The model under review builds one solid part; all positions refer to its coordinate system, in mm. Coordinates: 2 decimals unless noted, no trailing zeros. Order: outer loops, then holes, each group sorted by start corner. A loop starts at its lowest first (then second) coordinate and runs counter-clockwise, first axis right, second up.
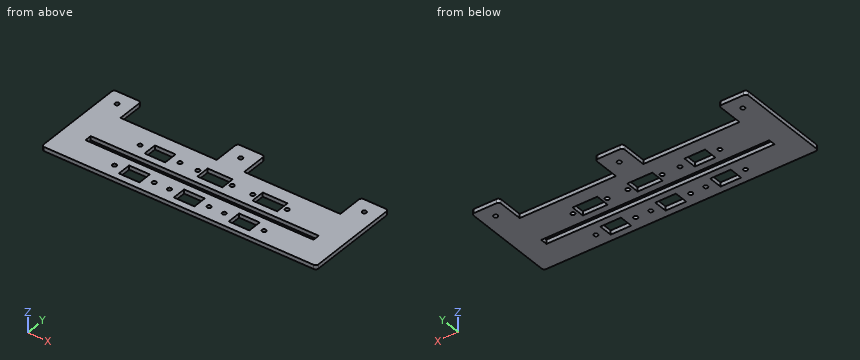
```python
from build123d import *

# Parameters (mm, degrees)
SKETCH_1_W           = 200
SKETCH_1_H           = 70
EXTRUDE_1_DEPTH      = 3
SKETCH_2_W           = 70
SKETCH_2_H           = 20
CUT_EXTRUDE_1_DEPTH  = 3
SKETCH_4_W           = 70
SKETCH_4_H           = 20
CUT_EXTRUDE_2_DEPTH  = 3
SKETCH_5_W           = 166
SKETCH_5_H           = 5
CUT_EXTRUDE_3_DEPTH  = 3
CUT_EXTRUDE_8_DEPTH  = 3
SKETCH_7_R           = 1.5
CUT_EXTRUDE_9_DEPTH  = 3
SKETCH_8_W           = 15
SKETCH_8_H           = 10
CUT_EXTRUDE_10_DEPTH = 3
SKETCH_9_W           = 15
SKETCH_9_H           = 10
SKETCH_9_W_2         = 18
SKETCH_9_W_3         = 18.2
CUT_EXTRUDE_11_DEPTH = 3
SKETCH_10_R          = 1.5
CUT_EXTRUDE_12_DEPTH = 3


with BuildPart() as part:
    # ｽｹｯﾁ1 → ﾎﾞｽ - 押し出し1 (new body)
    with BuildSketch(Plane.XY):
        Rectangle(SKETCH_1_W, SKETCH_1_H)
    extrude(amount=EXTRUDE_1_DEPTH)

    # ｽｹｯﾁ2 → ｶｯﾄ - 押し出し1 (cut)
    with BuildSketch(Plane.XY.offset(3)):
        with Locations((-45, 25)):
            Rectangle(SKETCH_2_W, SKETCH_2_H)
    extrude(amount=-CUT_EXTRUDE_1_DEPTH, mode=Mode.SUBTRACT)

    # ｽｹｯﾁ4 → ｶｯﾄ - 押し出し2 (cut)
    with BuildSketch(Plane.XY.offset(3)):
        with Locations((45, 25)):
            Rectangle(SKETCH_4_W, SKETCH_4_H)
    extrude(amount=-CUT_EXTRUDE_2_DEPTH, mode=Mode.SUBTRACT)

    # ｽｹｯﾁ5 → ｶｯﾄ - 押し出し3 (cut)
    with BuildSketch(Plane.XY.offset(3)):
        with Locations((0, -12.5)):
            Rectangle(SKETCH_5_W, SKETCH_5_H)
    extrude(amount=-CUT_EXTRUDE_3_DEPTH, mode=Mode.SUBTRACT)

    # ｽｹｯﾁ6 → ｶｯﾄ - 押し出し8 (cut)
    with BuildSketch(Plane.XY.offset(3)):
        with BuildLine():
            ThreePointArc((-98, -35), (-99.414213562, -34.414213562), (-100, -33))
            Line((-100, -33), (-100, -35))
            Line((-100, -35), (-98, -35))
        make_face()
        with BuildLine():
            Line((-100, 35), (-100, 33))
            ThreePointArc((-100, 33), (-99.414213562, 34.414213562), (-98, 35))
            Line((-98, 35), (-100, 35))
        make_face()
        with BuildLine():
            ThreePointArc((100, -33), (99.414213562, -34.414213562), (98, -35))
            Line((98, -35), (100, -35))
            Line((100, -35), (100, -33))
        make_face()
        with BuildLine():
            Line((-80, 35), (-82, 35))
            ThreePointArc((-82, 35), (-80.585786438, 34.414213562), (-80, 33))
            Line((-80, 33), (-80, 35))
        make_face()
        with BuildLine():
            ThreePointArc((98, 35), (99.414213562, 34.414213562), (100, 33))
            Line((100, 33), (100, 35))
            Line((100, 35), (98, 35))
        make_face()
        with BuildLine():
            ThreePointArc((80, 33), (80.585786438, 34.414213562), (82, 35))
            Line((82, 35), (80, 35))
            Line((80, 35), (80, 33))
        make_face()
        with BuildLine():
            Line((-10, 35), (-10, 33))
            ThreePointArc((-10, 33), (-9.414213562, 34.414213562), (-8, 35))
            Line((-8, 35), (-10, 35))
        make_face()
        with BuildLine():
            Line((10, 35), (8, 35))
            ThreePointArc((8, 35), (9.414213562, 34.414213562), (10, 33))
            Line((10, 33), (10, 35))
        make_face()
    extrude(amount=-CUT_EXTRUDE_8_DEPTH, mode=Mode.SUBTRACT)

    # ｽｹｯﾁ7 → ｶｯﾄ - 押し出し9 (cut)
    with BuildSketch(Plane.XY.offset(3)):
        with Locations((-90, 25)):
            Circle(SKETCH_7_R)
        with Locations((0, 25)):
            Circle(SKETCH_7_R)
        with Locations((90, 25)):
            Circle(SKETCH_7_R)
    extrude(amount=-CUT_EXTRUDE_9_DEPTH, mode=Mode.SUBTRACT)

    # ｽｹｯﾁ8 → ｶｯﾄ - 押し出し10 (cut)
    with BuildSketch(Plane.XY.offset(3)):
        with Locations((40, -25)):
            Rectangle(SKETCH_8_W, SKETCH_8_H)
        with Locations((0, -25)):
            Rectangle(SKETCH_8_W, SKETCH_8_H)
        with Locations((-40, -25)):
            Rectangle(SKETCH_8_W, SKETCH_8_H)
    extrude(amount=-CUT_EXTRUDE_10_DEPTH, mode=Mode.SUBTRACT)

    # ｽｹｯﾁ9 → ｶｯﾄ - 押し出し11 (cut)
    with BuildSketch(Plane.XY.offset(3)):
        with Locations((-40, 0)):
            Rectangle(SKETCH_9_W, SKETCH_9_H)
        with Locations((40, 0)):
            Rectangle(SKETCH_9_W_2, SKETCH_9_H)
        Rectangle(SKETCH_9_W_3, SKETCH_9_H)
    extrude(amount=-CUT_EXTRUDE_11_DEPTH, mode=Mode.SUBTRACT)

    # ｽｹｯﾁ10 → ｶｯﾄ - 押し出し12 (cut)
    with BuildSketch(Plane.XY.offset(3)):
        with Locations((-54.5, 0)):
            Circle(SKETCH_10_R)
        with Locations((-25.5, 0)):
            Circle(SKETCH_10_R)
        with Locations((-12.5, 0)):
            Circle(SKETCH_10_R)
        with Locations((12.5, 0)):
            Circle(SKETCH_10_R)
        with Locations((27.5, 0)):
            Circle(SKETCH_10_R)
        with Locations((52.5, 0)):
            Circle(SKETCH_10_R)
        with Locations((54.5, -25)):
            Circle(SKETCH_10_R)
        with Locations((25.5, -25)):
            Circle(SKETCH_10_R)
        with Locations((14.5, -25)):
            Circle(SKETCH_10_R)
        with Locations((-14.5, -25)):
            Circle(SKETCH_10_R)
        with Locations((-25.5, -25)):
            Circle(SKETCH_10_R)
        with Locations((-54.5, -25)):
            Circle(SKETCH_10_R)
    extrude(amount=-CUT_EXTRUDE_12_DEPTH, mode=Mode.SUBTRACT)


solid = part.part
```
(1) We need section C-C, the plane z = 0.7. Count the separate pieces of the cut face and the enclosed holes in it, and give its area (3 significant figures).
A:
separate pieces: 1
enclosed holes: 22
area: 9,300 mm2
(2) For pin 1 Ø1.8 at (x, y) = (-25.5, -25) entering from -Z, flat-tipped, find the tip position at first contact; note if it passes through.
A:
pin 1: passes through
(3) We need section B-B, the plane x = -20.5. Write out the cut boundary in (y, z), and give its area (3 significant figures).
A:
outline: (-35, 0) - (-15, 0) - (-15, 3) - (-35, 3) - close; (-10, 0) - (15, 0) - (15, 3) - (-10, 3) - close
area: 135 mm2
(4) We need section A-A, the plane y = 21.5. Write out the cut boundary in (x, z), and give its area (3 significant figures).
A:
outline: (-100, 0) - (-80, 0) - (-80, 3) - (-100, 3) - close; (-10, 0) - (10, 0) - (10, 3) - (-10, 3) - close; (80, 0) - (100, 0) - (100, 3) - (80, 3) - close
area: 180 mm2
(5) Wall thickness on probe 1 along X at (y, z) = (18, 0.75); probe 2 along X at (y, z) = (-22.5, 1.65); probe 3 along Y at (x, z) = (-14.5, 1.6): over which ranges is each line inside the solid? List them lowest first.
A:
probe 1: x = -100 to -80, -10 to 10, 80 to 100
probe 2: x = -100 to -47.5, -32.5 to -7.5, 7.5 to 32.5, 47.5 to 100
probe 3: y = -35 to -26.5, -23.5 to -15, -10 to 15
